```python
from build123d import *

# Parameters (mm, degrees)
EXTRUDE_1_DEPTH = 30


with BuildPart() as part:
    # 草图1 → 凸台-拉伸1 (new body)
    with BuildSketch(Plane.XY):
        Polygon((25, -14.43375673), (25, 14.43375673), (0, 28.867513459), (-25, 14.43375673), (-25, -14.43375673), (0, -28.867513459), align=None)
    extrude(amount=EXTRUDE_1_DEPTH)

    # 草图2 → 切除-旋转1 (revolve, cut)
    with BuildSketch(Plane(origin=(0, 0, 0), x_dir=(0, 0, -1), z_dir=(1, 0, 0)), mode=Mode.PRIVATE) as cut_revolve_1_sk:
        Polygon((-4, 28.908520158), (0.613826619, 20.917138036), (0.613826619, 32.83436024), align=None)
    revolve(cut_revolve_1_sk.sketch.rotate(Axis((0, 0, -10.704078941), (0, 0, 1)), 270), axis=Axis((0, 0, -10.704078941), (0, 0, 1)), mode=Mode.SUBTRACT)


solid = part.part
```
Geometry: final body of the model. Coordinates: model frame, mm. Coordinates: 2 decimals unless noted, no trailing zeros. Order: outer loops, then holes, each group sorted by start corner. A loop starts at its lowest first (then second) coordinate and runs counter-clockwise, first axis right, second up. Notation, with made-up numbers: M 79,-1.75 L 85,-1.75 A20 cw 85,33.25 Z; hole C -29.5,65 d5. An arc over 180 degrees is marked long. Answer as CSV lines item,"result".
Q1. Line query: probe 1 along Z at (x, y) = (-2, 23.5); probe 2 along Y at (x, z) = (1, 25.5); probe 3 along Y at (x, z) = (-7, 27.75). Output: solid intervals per line, ascending. Write a range as [from, to].
Answers:
probe 1,"z = [0.93, 30]"
probe 2,"y = [-28.29, 28.29]"
probe 3,"y = [-24.83, 24.83]"
Q2. Section A-A on z = 9.25. Return the cut outline in (x, y), and give its area (3 significant figures).
Answers:
outline,"M -25,-14.43 L 0,-28.87 L 25,-14.43 L 25,14.43 L 0,28.87 L -25,14.43 Z"
area,"2,170 mm^2"
Q3. First-contact query: P1, Ø1.5, axis at x = -3, z = 14.5, coming from the +Y side; P2, Ø5, axis at x = -7, z = 15.5, coming from the -Y side; P3, Ø1, axis at x = 3, z = 14, coming from the -Y side. Flat tips, straight axial feed; report the tip coordinate or a pass-through.
Answers:
P1,"stops at y = 27.57"
P2,"stops at y = -26.27"
P3,"stops at y = -27.42"
